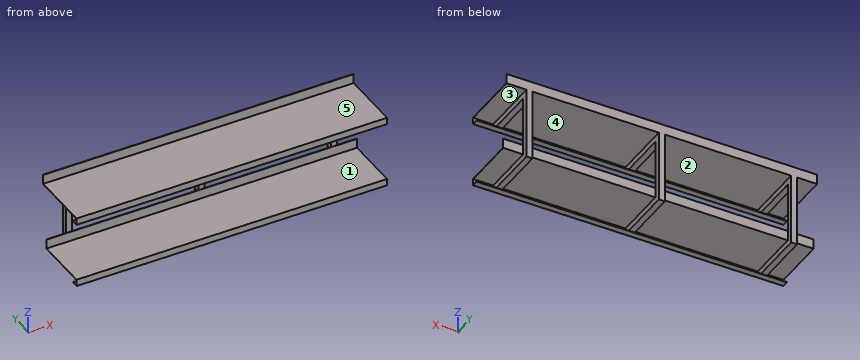
from build123d import *

# Parameters (mm, degrees)
F1_DEPTH      = 30
F5_DEPTH      = 30
F7_DEPTH      = 15
F7_DEPTH_BACK = 15
F9_DEPTH      = 780
F9_DEPTH_BACK = 780


with BuildPart() as f1:
    # F0 (on Right) → F1 (new body)
    with BuildSketch(Plane.YZ):
        Polygon((0, 30), (0, 0), (300, 0), (300, 360), (0, 360), (0, 330), (270, 330), (270, 30), align=None)
    extrude(amount=F1_DEPTH)



with BuildPart() as f5:
    # F4 (on offset) → F5 (new body)
    with BuildSketch(Plane.YZ.offset(1360)):
        Polygon((0, 30), (0, 0), (300, 0), (300, 360), (0, 360), (0, 330), (270, 330), (270, 30), align=None)
    extrude(amount=-F5_DEPTH)


with BuildPart() as f7:
    # F6 (on mid) → F7 (new body, two sides)
    with BuildSketch(Plane.YZ.offset(680)) as f7_sk:
        Polygon((0, 30), (0, 0), (300, 0), (300, 360), (0, 360), (0, 330), (270, 330), (270, 30), align=None)
    extrude(amount=F7_DEPTH)
    extrude(f7_sk.sketch, amount=-F7_DEPTH_BACK)


with BuildPart() as f1_1:
    add(f1.part)

    add(f5.part)  # F9 merges F5

    add(f7.part)  # F9 merges F7
    # F8 (on mid) → F9 (join, two sides)
    with BuildSketch(Plane.YZ.offset(680)) as f9_sk:
        Polygon((30, 0), (0, 0), (0, 30), (270, 30), (270, 80), (268, 80), (268, 32), (-2, 32), (-2, -2), (30, -2), align=None)
        Polygon((30, 330), (0, 330), (0, 360), (300, 360), (300, 410), (298, 410), (298, 362), (-2, 362), (-2, 328), (30, 328), align=None)
    extrude(amount=F9_DEPTH)
    extrude(f9_sk.sketch, amount=-F9_DEPTH_BACK)


solid = f1_1.part
Work out the finished part from the listing and answer in its coordinate system (mm). Face numbers are marked on the shaded views. A direction names the side the tool comes from. Round coordinates to 2 decimals unless told otherwise and drop trailing zeros. Loops run counter-clockwise (first coordinate to the right, second up) from the corner with the lowest first, then second, coordinate; pieces in that order, holes last. Notation, with made-up numbers: M -15,2 L 23,2 A28 cw 23,27 Z; hole C 82.25,18 d5. An arc over 180 degrees is marked long. One line per question, with ' | ' between items. Start each with the question number.
(1) For a pull along Z with two mould halves and no side action, classify the marked faces 4 and 5 as released by +Z, released by -Z, zero draft, split by the parting line, or undercut.
(2) A cutting plane is placed at B-B on x = 1216. Write down the section's boundary in (y, z), plus the area to 3 significant figures.
(3) Flat-ended cylindrical pins translate along their axes: pin 1 Ø15 at (x, z) = (1146.5, 43.5) entering from +Y; pin 2 Ø24 at (x, y) = (9, 98) entering from -Z; pin 3 Ø1.6 at (x, z) = (946.5, 329) entering from +Y. Find the tip coordinate at first contact, or state that the pin passes through.
(4) A cutting plane is placed at A-A on z = 260. Write down the section's boundary in (x, y).
(5) Find the intervals of material crossed by line 1 (X direction, y = 260, z = 21); line 2 (Z direction, x = -15, y = 214.5); line 3 (Z direction, x = 1332, y = 113), in increasing order.
(6) A tool of negligible diameter and unlimited length cuts with its end or side. For the marked faces 1, 2 and 3, from which of +Z, -Z, +X, -X, +Y, -Y can it reach the whole face along a straight path? Write none if from no direction.
Geometry check:
1) face 4: undercut | face 5: released by +Z
2) outline: M -2,-2 L 30,-2 L 30,0 L 0,0 L 0,30 L 270,30 L 270,80 L 268,80 L 268,32 L -2,32 Z; M -2,328 L 30,328 L 30,330 L 0,330 L 0,360 L 300,360 L 300,410 L 298,410 L 298,362 L -2,362 Z | area: 1,590 mm²
3) pin 1: stops at y = 270 | pin 2: stops at z = 0 | pin 3: stops at y = 30
4) outline: M 0,270 L 30,270 L 30,300 L 0,300 Z; M 665,270 L 695,270 L 695,300 L 665,300 Z; M 1330,270 L 1360,270 L 1360,300 L 1330,300 Z
5) line 1: x = 0 to 30, 665 to 695, 1330 to 1360 | line 2: z = 30 to 32, 360 to 362 | line 3: z = 0 to 32, 330 to 362
6) face 1: +X, -X, -Y | face 2: +Y | face 3: +X, +Y
